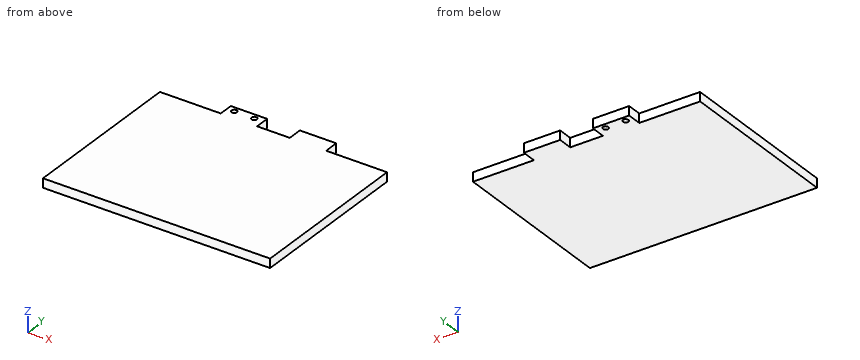
```python
from build123d import *

# Parameters (mm, degrees)
RESSALTO_EXTRUS_O1_DEPTH = 5
ESBO_O2_R                = 1.5
CORTE_EXTRUS_O1_DEPTH    = 10


with BuildPart() as part:
    # Esboço1 → Ressalto-extrusão1 (new body)
    with BuildSketch(Plane.XY):
        Polygon((-1.556986729, 38.142857143), (16.443013271, 38.142857143), (16.443013271, 46.142857143), (36.443013271, 46.142857143), (36.443013271, 38.142857143), (69.943013271, 38.142857143), (69.943013271, -54.857142857), (-55.056986729, -54.857142857), (-55.056986729, 38.142857143), (-21.556986729, 38.142857143), (-21.556986729, 46.142857143), (-1.556986729, 46.142857143), align=None)
    extrude(amount=RESSALTO_EXTRUS_O1_DEPTH)

    # Esboço2 → Corte-extrusão1 (cut)
    with BuildSketch(Plane.XY.offset(5)):
        with Locations((-17.556986729, 43.142857143)):
            Circle(ESBO_O2_R)
        with Locations((-6.556986729, 43.142857143)):
            Circle(ESBO_O2_R)
    extrude(amount=-CORTE_EXTRUS_O1_DEPTH, mode=Mode.SUBTRACT)


solid = part.part
```
Could you check a few things on this model? Use its own coordinates, in mm. Round coordinates to 2 decimals unless told otherwise and drop trailing zeros. Loops run counter-clockwise (first coordinate to the right, second up) from the corner with the lowest first, then second, coordinate; pieces in that order, holes last. Notation, with made-up numbers: (82.5, -18.5) - (98.5, -18.5) arc R26 ccw to (98.5, 16.5) - close; hole circle Ø7 at (72, -16.5). An arc over 180 degrees is marked (long way). Answer in a Markdown table with one row per item. Add a question column.
(1) I'm going to push flat-ended pins straight in: pin 1 (2.5 mm diameter, centred on x = 58, z = 1.5, fed in from +Y); pin 2 (2.5 mm diameter, centred on y = 42, z = 3, fed in from +X); pin 3 (2.5 mm diameter, centred on y = 44, z = 2.5, fed in from -X). Where does each tip first touch, or does it pass through?
(2) If we section it at A-A (z = 3.15): Please give me the cut outline in (x, y).
(3) I need wall thicknesses on line 1 along X through (y, z) = (39.5, 1.05); line 2 along Y through (x, z) = (59.5, 2.15). Which ranges of each line are inside material? Lowest first, please.
(4) If we section it at B-B (x = -43.5): Please give me the cut outline in (y, z).
Model answer:
| question | item | result |
|---|---|---|
| 1 | pin 1 | stops at y = 38.14 |
| 1 | pin 2 | stops at x = 36.44 |
| 1 | pin 3 | stops at x = -21.56 |
| 2 | outline | (-55.06, -54.86) - (69.94, -54.86) - (69.94, 38.14) - (36.44, 38.14) - (36.44, 46.14) - (16.44, 46.14) - (16.44, 38.14) - (-1.56, 38.14) - (-1.56, 46.14) - (-21.56, 46.14) - (-21.56, 38.14) - (-55.06, 38.14) - close; hole circle Ø3 at (-17.56, 43.14); hole circle Ø3 at (-6.56, 43.14) |
| 3 | line 1 | x = -21.56 to -1.56, 16.44 to 36.44 |
| 3 | line 2 | y = -54.86 to 38.14 |
| 4 | outline | (-54.86, 0) - (38.14, 0) - (38.14, 5) - (-54.86, 5) - close |
